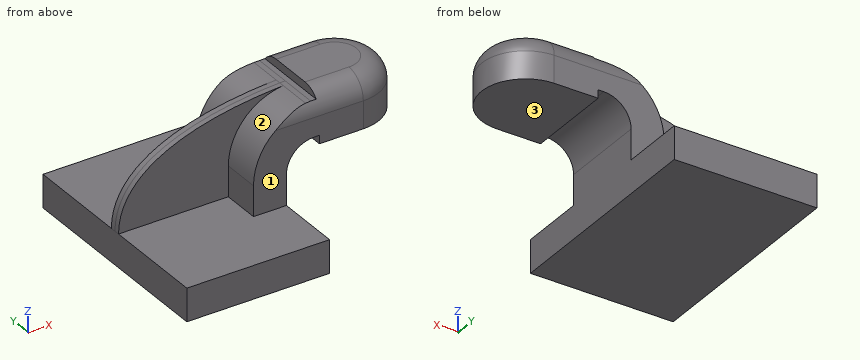
```python
from build123d import *

# Parameters (mm, degrees)
F1_DEPTH = 63.5
F0_W     = 25.4
F0_H     = 19.05
F0_H_2   = 4.7498
F0_H_3   = 4.7752
F2_DEPTH = 25.4
F4_DEPTH = 3.175
F5_R     = 12.7


with BuildPart() as f1:
    # F0 (on Front) → F1 (new body, symmetric)
    with BuildSketch(Plane.XZ):
        Polygon((41.275, -9.525), (41.275, 9.525), (22.225, 9.525), (-41.275, 9.525), (-41.275, -9.525), align=None)
    extrude(amount=F1_DEPTH, both=True)

    # F0 (on Front) → F2 (join, symmetric)
    with BuildSketch(Plane.XZ):
        with BuildLine():
            Line((22.225, 9.525), (41.275, 9.525))
            Line((41.275, 9.525), (41.275, 27.0002))
            ThreePointArc((41.275, 27.0002), (45.9246798487, 38.2255201513), (57.15, 42.8752))
            Line((57.15, 42.8752), (60.325, 42.8752))
            Line((60.325, 42.8752), (60.325, 61.9252))
            Line((60.325, 61.9252), (57.15, 61.9252))
            add(Edge.make_bspline(
                [(54.0587441636, 61.7881255253), (55.0869767217, 61.838850256), (56.1175065912, 61.8845174455), (57.15, 61.9252)],
                knots=[109.2703067259, 109.2703067259, 109.2703067259, 109.2703067259, 111.5045361635, 111.5045361635, 111.5045361635, 111.5045361635], degree=3))
            ThreePointArc((54.0587441636, 61.7881255253), (31.3845411928, 50.5776629139), (22.225, 27.0002))
            Line((22.225, 27.0002), (22.225, 9.525))
        make_face()
        with Locations((73.025, 52.4002)):
            Rectangle(F0_W, F0_H)
        with Locations((73.025, 64.3001)):
            Rectangle(F0_W, F0_H_2)
        with Locations((73.025, 40.4876)):
            Rectangle(F0_W, F0_H_3)
    extrude(amount=F2_DEPTH, both=True)

    # F0 (on Front) → F3 (revolve)
    with BuildSketch(Plane.XZ):
        Polygon((85.725, 61.9252), (85.725, 42.8752), (85.725, 38.1), (111.125, 38.1), (111.125, 66.675), (85.725, 66.675), align=None)
    revolve(axis=Axis((85.725, 0, 52.3875), (0, 0, 1)))

    # F0 (on Front) → F4 (join, symmetric)
    with BuildSketch(Plane.XZ):
        with BuildLine():
            Line((-41.275, 9.525), (22.225, 9.525))
            Line((22.225, 9.525), (22.225, 27.0002))
            ThreePointArc((22.225, 27.0002), (31.3845411928, 50.5776629139), (54.0587441636, 61.7881255253))
            add(Edge.make_bspline(
                [(-41.275, 9.525), (-41.0225634855, 44.7292047169), (3.7705843511, 59.3073118764), (54.0587441636, 61.7881255253)],
                knots=[0, 0, 0, 0, 109.2703067259, 109.2703067259, 109.2703067259, 109.2703067259], degree=3))
        make_face()
    extrude(amount=F4_DEPTH, both=True)

    # F5
    f5_edges = [f1.edges().sort_by_distance(p)[0] for p in [
        (85.725, 25.4, 52.3875),
        (73.025, 25.4, 66.675),
        (73.025, -25.4, 66.675),
        (111.125, 0, 66.675),
    ]]
    fillet(f5_edges, radius=F5_R)


solid = f1.part
```
Model file for the job. Use its own axes, mm. Face numbers are marked on the shaded views. A direction names the side the tool comes from. Give positions to 0.01 mm unless a question says otherwise; leave off trailing zeros. Loops run counter-clockwise (first coordinate to the right, second up) from the corner with the lowest first, then second, coordinate; pieces in that order, holes last. Notation, with made-up numbers: (4, -34) - (47, -34) arc R20 ccw to (47, -22) - close; hole circle Ø7 at (0.25, 30). An arc over 180 degrees is marked (long way). One line per item, written item: value. Start each with the question number.
1. Slice it at A-A (z = 3.5). List the corners of the cut face in (x, y) (3 decimals), plus the area to 3 significant figures.
2. Pin check, flat tips, straight feed: pin 1 (2.5 mm diameter, centred on y = -3.5, z = 40.5, fed in from -X); pin 2 (4 mm diameter, centred on y = -10, z = 57.5, fed in from -X); pin 3 (5 mm diameter, centred on y = 13, z = 20.5, fed in from -X) (3 decimals). Stop position of each tip, or through.
3. Probe L1, parallel to Z at x = -30, y = 44.5 (3 decimals); L2, parallel to Y at x = -23, z = 37.5 (3 decimals); L3, parallel to Z at x = 67.5, y = 0 (3 decimals). List the from-to ranges inside material, lowest first. Write a range as from..to.
4. Which spindle directions (+Z, -Z, +X, -X, +Y, -Y) get a long thin tool onto all of the face, cutting with end or side? Do the marked faces 1, 2 and 3. Say none if no direction does.
5. Slice it at B-B (y = 43). List the corners of the cut face in (x, z) (3 decimals).
Solution:
1. outline: (-41.275, -63.5) - (41.275, -63.5) - (41.275, 63.5) - (-41.275, 63.5) - close
1. area: 10,500 mm^2
2. pin 1: stops at x = -26.29
2. pin 2: stops at x = 36.96
2. pin 3: stops at x = 22.225
3. L1: z = -9.525..9.525
3. L2: y = -3.175..3.175
3. L3: z = 38.1..66.675
4. face 1: +Z, +X, -X, -Y
4. face 2: +Z, -X, -Y
4. face 3: -Z, +X, +Y, -Y
5. outline: (-41.275, -9.525) - (41.275, -9.525) - (41.275, 9.525) - (-41.275, 9.525) - close
